The figure shows three views and two pictorial views of one solid part (mm, origin at its lowest corner). Answer the questions. Coordinates: 2 decimals unless noted, no trailing zeros. Loops run counter-clockwise (first coordinate to the right, second up) from the corner with the lowest first, then second, coordinate; pieces in that order, holes last.
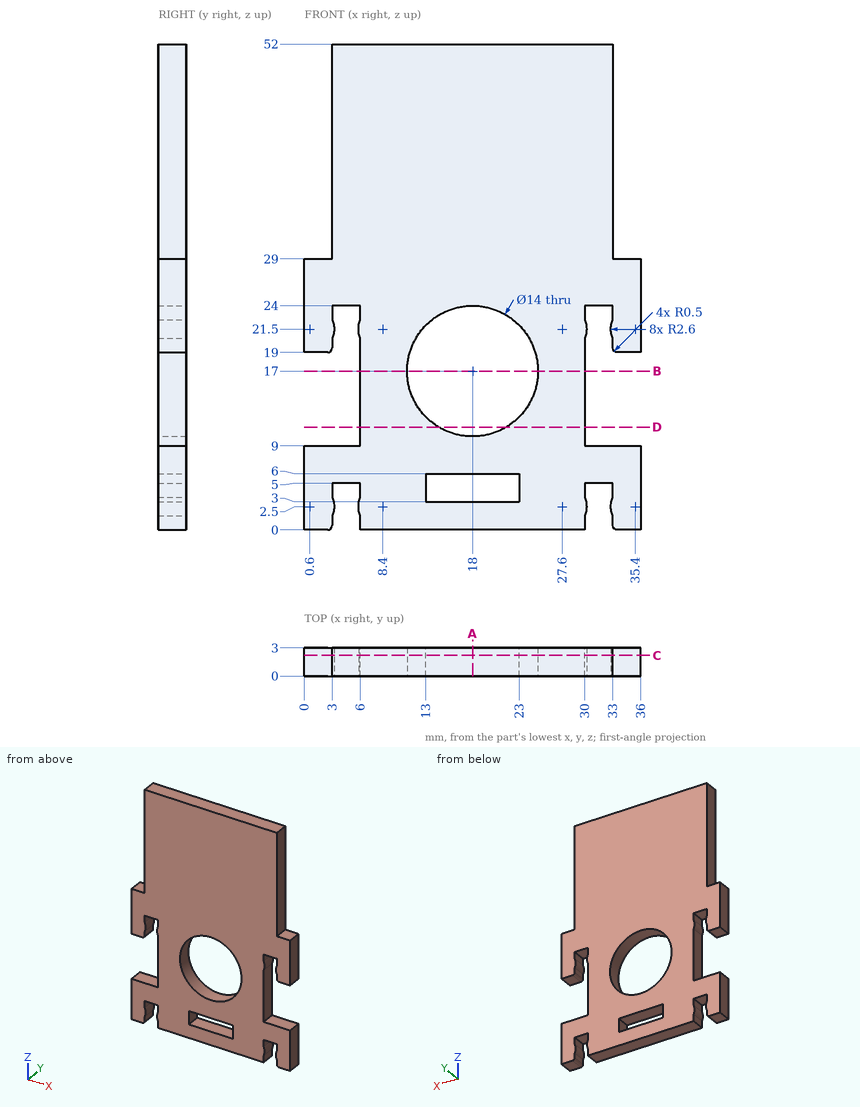
Q1. A cutting plane is placed at D-D (z = 11). Give the vertices of the cut face in (x, y).
Findings below:
outline: (6, 0) - (14.39, 0) - (14.39, 3) - (6, 3) - close; (21.61, 0) - (30, 0) - (30, 3) - (21.61, 3) - close
Q2. Flat-ended cylindrical pins translate along their axes: pin 1 Ø0.9 at (x, y) = (31.5, 1) entering from -Z; pin 2 Ø0.9 at (y, z) = (1, 40.5) entering from +X. Find the tip coordinate at first contact, or state that the pin passes through.
Findings below:
pin 1: stops at z = 5
pin 2: stops at x = 33
Q3. Straight lines are drawn through the part: probe 1 along X at (y, z) = (2.25, 2.5); probe 2 along Z at (x, y) = (32.5, 1.85); probe 3 along X at (y, z) = (0.7, 17). For each, find the intervals that lie inside material, in ascending order.
Findings below:
probe 1: x = 0 to 3.2, 5.8 to 30.2, 32.8 to 36
probe 2: z = 5 to 9, 24 to 52
probe 3: x = 6 to 11, 25 to 30
Q4. A cutting plane is placed at B-B (z = 17). Give the vertices of the cut face in (x, y).
Findings below:
outline: (6, 0) - (11, 0) - (11, 3) - (6, 3) - close; (25, 0) - (30, 0) - (30, 3) - (25, 3) - close
Q5. A cutting plane is placed at C-C (y = 2.2). Count the separate pieces of the cut face and the enclosed holes in it, then the cut area to 3 significant figures.
Findings below:
separate pieces: 1
enclosed holes: 2
area: 1,370 mm2
Q6. A cutting plane is placed at A-A (x = 18). Give the vertices of the cut face in (y, z).
Findings below:
outline: (0, 0) - (3, 0) - (3, 3) - (0, 3) - close; (0, 6) - (3, 6) - (3, 10) - (0, 10) - close; (0, 24) - (3, 24) - (3, 52) - (0, 52) - close
